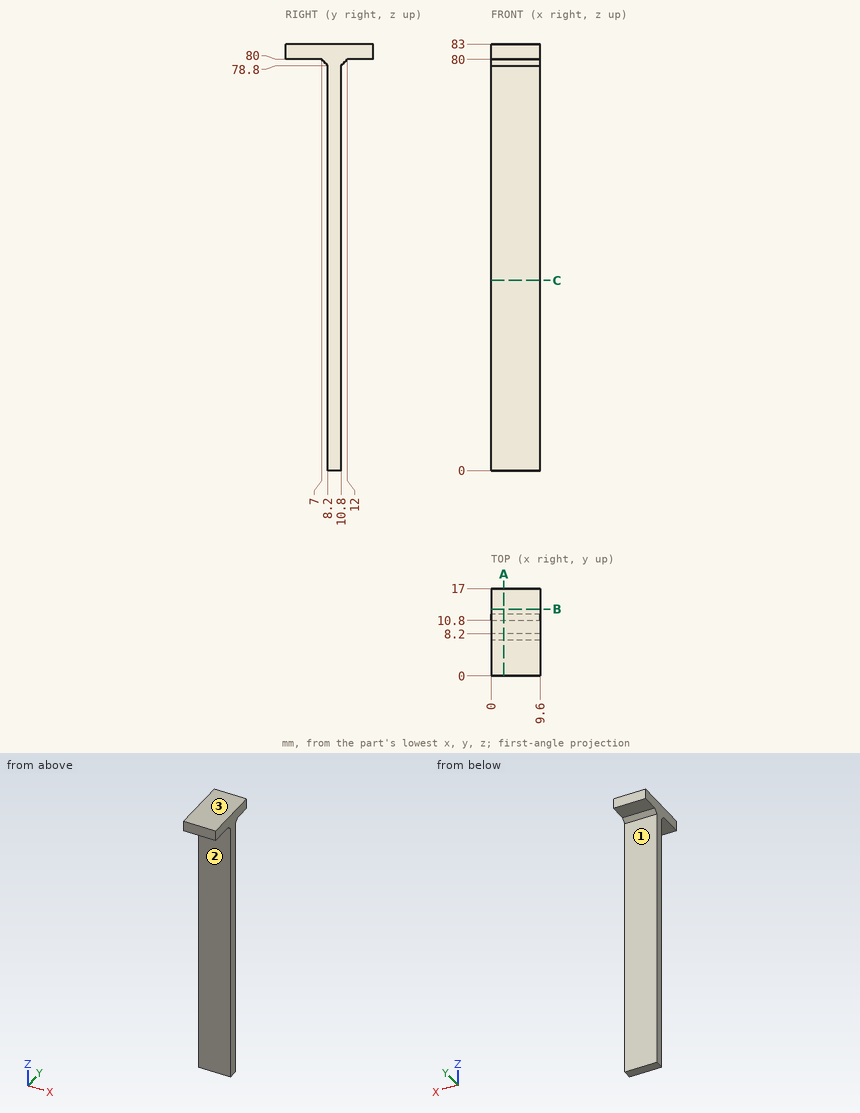
Drawing for the job (mm, zero at the part's lowest x, y, z). A direction names the side the tool comes from. Round coordinates to 2 decimals unless told otherwise and drop trailing zeros. Order: outer loops, then holes, each group sorted by start corner. A loop starts at its lowest first (then second) coordinate and runs counter-clockwise, first axis right, second up.
Item 1: Saw through at C-C on z = 37. Write the cut outline in (x, y), then the cut area to 3 significant figures.
Item 2: Saw through at A-A on x = 2.5. Write the cut outline in (y, z).
Item 3: Probe line 1 along Y through (x, z) = (1, 74); line 2 along Z through (x, y) = (6, 16.25); line 3 along Z through (x, y) = (3.75, 11.25). List the from-to ranges inside material, lowest first.
Item 4: Saw through at B-B on y = 13. Write the cut outline in (x, z), then the cut area to 3 significant figures.
Item 5: Pin check, flat tips, straight feed: pin 1 (3 mm diameter, centred on x = 4.5, z = 34.5, fed in from +Y); pin 2 (3 mm diameter, centred on x = 6.5, z = 40.5, fed in from -Y); pin 3 (3.5 mm diameter, centred on x = 6.5, y = 2, fed in from -Z); pin 4 (8 mm diameter, centred on y = 4.5, z = 43, fed in from -X). Stop position of each tip, or through.
Item 6: Tool access for the marked faces 1, 2 and 3: list every direction of +Z, -Z, +X, -X, +Y, -Y with a clear straight run to the whole face (end or side of a thin tool).
Reported:
1. outline: (0, 8.2) - (9.6, 8.2) - (9.6, 10.8) - (0, 10.8) - close
1. area: 25.0 mm2
2. outline: (0, 80) - (7, 80) - (8.2, 78.8) - (8.2, 0) - (10.8, 0) - (10.8, 78.8) - (12, 80) - (17, 80) - (17, 83) - (0, 83) - close
3. line 1: y = 8.2 to 10.8
3. line 2: z = 80 to 83
3. line 3: z = 79.25 to 83
4. outline: (0, 80) - (9.6, 80) - (9.6, 83) - (0, 83) - close
4. area: 28.8 mm2
5. pin 1: stops at y = 10.8
5. pin 2: stops at y = 8.2
5. pin 3: stops at z = 80
5. pin 4: stops at x = 0
6. face 1: -Z, +X, -X, +Y
6. face 2: -Z, +X, -X, -Y
6. face 3: +Z, +X, -X, +Y, -Y
